Model file for the job. Use its own axes, mm. Face numbers are marked on the shaded views. Round coordinates to 2 decimals unless told otherwise and drop trailing zeros. Loops run counter-clockwise (first coordinate to the right, second up) from the corner with the lowest first, then second, coordinate; pieces in that order, holes last.
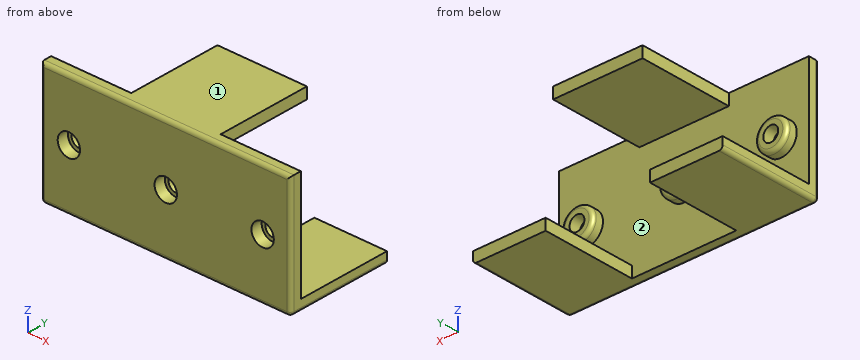
Autodesk Inventor part; units mm, degrees
ref_plane "YZ Plane" through (0, 0, 0) normal (1, 0, 0) x (0, 1, 0)
ref_plane "XZ Plane" through (0, 0, 0) normal (0, 1, 0) x (-1, 0, 0)
ref_plane "XY Plane" through (0, 0, 0) normal (0, 0, 1) x (1, 0, 0)
sketch "Sketch1" plane through (0, 0, 0) normal (0, 1, 0) x (-1, 0, 0)
  line L0 (20.5, 16.2) -> (-20.5, 16.2)
  line L1 (-20.5, 16.2) -> (-20.5, -16.2)
  line L2 (-20.5, -16.2) -> (20.5, -16.2)
  line L3 (20.5, -16.2) -> (20.5, 16.2)
  point P0 (0, 0)
  dimension "d0" = 41
  dimension "d1" = 32.4
extrude "Extrusion1" add sketch "Sketch1" along normal blind 3
sketch "Sketch3" plane through (0, 3, 0) normal (0, 1, 0) x (1, 0, 0)
  line L0 (-20.5, -16.2) -> (20.5, -16.2)
  line L1 (-20.5, 16.2) -> (-20.5, -16.2)
  line L2 (20.5, -16.2) -> (-20.5, -16.2)
  line L3 (-20.5, -16.2) -> (-20.5, -13.2)
  line L4 (-20.5, -13.2) -> (20.5, -13.2)
  line L5 (20.5, -13.2) -> (20.5, -16.2)
  line L6 (20.5, 16.2) -> (-20.5, 16.2)
  line L7 (20.5, 16.2) -> (-20.5, 16.2)
  line L8 (-20.5, 16.2) -> (-20.5, 13.2)
  line L9 (-20.5, 13.2) -> (20.5, 13.2)
  line L10 (20.5, 13.2) -> (20.5, 16.2)
  point P0 (0, 0)
  dimension "d8" = 3
  dimension "d9" = 3
extrude "Extrusion3" add sketch "Sketch3" along normal blind 25.4
sketch "Sketch4" plane through (20.5, 0, -16.2) normal (0, 0, -1) x (-1, 0, 0)
  line L0 (41, 3) -> (0, 3)
  line L1 (0, 28.4) -> (41, 28.4)
  line L2 (0, 3) -> (21.5, 3)
  line L3 (21.5, 3) -> (21.5, 28.4)
  line L4 (21.5, 28.4) -> (0, 28.4)
  line L5 (0, 28.4) -> (0, 3)
  point P0 (20.5, 0)
  dimension "d12" = 21.5
extrude "Extrusion4" cut sketch "Sketch4" against normal blind 3
sketch "Sketch5" plane through (-20.5, 0, 16.2) normal (0, 0, 1) x (1, 0, 0)
  line L0 (41, 28.4) -> (0, 28.4)
  line L1 (19.5, 3) -> (41, 3)
  line L2 (0, 28.4) -> (21.5, 28.4)
  line L3 (21.5, 28.4) -> (21.5, 3)
  line L4 (21.5, 3) -> (0, 3)
  line L5 (0, 3) -> (0, 28.4)
  point P0 (20.5, 0)
  dimension "d15" = 21.5
extrude "Extrusion5" cut sketch "Sketch5" against normal blind 3
sketch "Sketch6" plane through (0, 3, 0) normal (0, 1, 0) x (1, 0, 0)
  circle A0 centre (13, 0) radius 4.25
  circle A1 centre (-13, 0) radius 4.25
  line L0 (-20.5, 13.2) -> (-20.5, -16.2)
  line L1 (20.5, -13.2) -> (20.5, 16.2)
  point P0 (0, 0)
  dimension "d20" = 8.5
  dimension "d21" = 8.5
  dimension "d32" = 26
  dimension "d33" = 7.5
  dimension "d34" = 7.5
extrude "Extrusion6" add sketch "Sketch6" along normal blind 3
sketch "Sketch9" plane through (20.5, 0, 16.2) normal (1, 0, 0) x (0, 0, -1)
  line L0 (32.4, 0) -> (32.4, 3)
  line L1 (32.4, 3) -> (0, 3)
  line L2 (0, 3) -> (0, 0)
  line L3 (0, 0) -> (32.4, 0)
  line L4 (32.4, 0) -> (32.4, 3)
  point P0 (16.2, 0)
extrude "Extrusion9" add sketch "Sketch9" along normal blind 26
sketch "Sketch10" plane through (0, 3, 0) normal (0, 1, 0) x (1, 0, 0)
  circle A0 centre (39, 0) radius 4.25
  point P0 (0, 0)
  dimension "d37" = 8.5
extrude "Extrusion10" add sketch "Sketch10" along normal blind 3
sketch "Sketch11" plane through (0, 3, 0) normal (0, 1, 0) x (1, 0, 0)
  line L0 (46.5, 16.2) -> (46.5, -16.2)
  line L1 (46.5, 16.2) -> (27, 16.2)
  line L2 (27, 16.2) -> (27, 13.2)
  line L3 (27, 13.2) -> (46.5, 13.2)
  line L4 (46.5, 13.2) -> (46.5, 16.2)
  point P0 (0, 0)
  dimension "d40" = 19.5
  dimension "d41" = 3
extrude "Extrusion11" add sketch "Sketch11" along normal blind 25.4
sketch "Sketch14" plane through (20.5, 3, 13.2) normal (1, 0, 0) x (0, 0, -1)
  line L0 (0, 0) -> (0, 25.4)
  line L1 (-3, 0) -> (-3, 25.4)
  line L2 (0, 25.4) -> (-3, 25.4)
  line L3 (-3, 25.4) -> (-3, 0)
  line L4 (-3, 0) -> (0, 0)
  line L5 (0, 0) -> (0, 25.4)
  point P0 (13.2, -3)
extrude "Extrusion14" add sketch "Sketch14" along normal blind 4.5
fillet "Fillet1" radius 1 3 edges at (-17.25, 6, 0) (8.75, 6, 0) (34.75, 6, 0)
fillet "Fillet2" radius 1 6 edges at (-20.5, 14.2, -16.2) (-20.5, 0, 0) (13, 0, 16.2) (46.5, 0, 0) (46.5, 14.2, -16.2) (13, 0, -16.2)
sketch "Sketch15" plane through (0, 0, 0) normal (0, -1, 0) x (1, 0, 0)
  circle A0 centre (39, 0) radius 4.25
  circle A1 centre (39, 0) radius 2
  circle A2 centre (13, 0) radius 3.25
  circle A3 centre (13, 0) radius 2
  circle A4 centre (-13, 0) radius 3.25
  circle A5 centre (-13, 0) radius 2
  point P0 (0, 0)
  dimension "d54" = 4
  dimension "d55" = 4
  dimension "d56" = 4
extrude "Extrusion15" cut sketch "Sketch15" against normal blind 10 contours A1 | A3 | A5
sketch "Sketch16" plane through (0, 0, 0) normal (0, -1, 0) x (1, 0, 0)
  circle A0 centre (39, 0) radius 2
  circle A1 centre (39, 0) radius 3
  circle A2 centre (13, 0) radius 2
  circle A3 centre (13, 0) radius 3
  circle A4 centre (-13, 0) radius 2
  circle A5 centre (-13, 0) radius 3
  point P0 (0, 0)
  dimension "d59" = 6
  dimension "d60" = 6
  dimension "d61" = 6
extrude "Extrusion16" cut sketch "Sketch16" against normal blind 3 contours A0 | A1 | A2 | A3 | A4 | A5
properties part number "railBracketBottom"
Q1. Slice it at B-B on y = 9. Give the cut face in (x, z).
Q2. Slice it at C-C on y = 2. Give the cut face in (x, z).
Q3. Flat gauge pins, fed straight in: P1, Ø7, axis at x = 37.5, z = -1.5, coming from the +Y side; P2, Ø3.5, axis at y = 14, z = 15, coming from the +X side; P3, Ø10, axis at x = -9, y = 11.5, coming from the +Z side. Where does each tip first touch, or does it go through?
Q4. Probe line 1 (Z direction, x = 39, y = 5); line 2 (Z direction, x = 13, y = 1.05); line 3 (Y direction, x = 30, z = 0.5). List the from-to ranges inside material, lowest first.
Q5. Slice it at D-D on z = 0. State how many separate pieces and enclosed holes the cut face has, plus the area to 3 significant figures.
Q6. Pull direction X, two halves, no side cores. Call the marked faces 1 and 2: pulls with the +X half, pulls with the -X half, needs draft (parallel to the pull), parting line crosses it, or undercut.
Q7. Slice it at A-A on x = 39. Give the cut face in (y, z), plus the area to 3 significant figures.
Reply:
1. outline: (-20.5, -15.2) arc R1 ccw to (-19.5, -16.2) - (-1, -16.2) - (-1, -13.2) - (-20.5, -13.2) - close; (1, 13.2) - (25, 13.2) - (25, 16.2) - (1, 16.2) - close; (27, -16.2) - (45.5, -16.2) arc R1 ccw to (46.5, -15.2) - (46.5, -13.2) - (27, -13.2) - close
2. outline: (-20.5, -15.2) arc R1 ccw to (-19.5, -16.2) - (45.5, -16.2) arc R1 ccw to (46.5, -15.2) - (46.5, 16.2) - (-20.5, 16.2) - close; hole circle Ø6 at (-13, 0); hole circle Ø6 at (13, 0); hole circle Ø6 at (39, 0)
3. P1: stops at y = 6
3. P2: stops at x = 25
3. P3: stops at z = -13.2
4. line 1: z = -16.2 to -13.2, -4.25 to -2, 2 to 4.25
4. line 2: z = -16.2 to -3, 3 to 16.2
4. line 3: y = 0 to 3
5. separate pieces: 4
5. enclosed holes: 0
5. area: 186 mm2
6. face 1: needs draft
6. face 2: undercut
7. outline: (0, -15.2) arc R1 ccw to (1, -16.2) - (28.4, -16.2) - (28.4, -13.2) - (3, -13.2) - (3, -4.25) - (5, -4.25) arc R1 ccw to (6, -3.25) - (6, -2) - (3, -2) - (3, -3) - (0, -3) - close; (0, 3) - (3, 3) - (3, 2) - (6, 2) - (6, 3.25) arc R1 ccw to (5, 4.25) - (3, 4.25) - (3, 16.2) - (1, 16.2) arc R1 ccw to (0, 15.2) - close
7. area: 168 mm2
